from build123d import *

# Parameters (mm, degrees)
F0_W     = 30
F0_H     = 30
F1_DEPTH = 30
F2_R     = 25
F3_DEPTH = 1
F4_R     = 25
F4_R_2   = 15
F5_DEPTH = 30


with BuildPart() as f1:
    # F0 (on Top) → F1 (new body)
    with BuildSketch(Plane.XY):
        Rectangle(F0_W, F0_H)
    extrude(amount=F1_DEPTH)

    # F2 (on face) → F3 (join)
    with BuildSketch(Plane(origin=(0, 0, 0), x_dir=(1, 0, 0), z_dir=(0, 0, -1))):
        Circle(F2_R)
        Polygon((15, 15), (15, 0), (15, -15), (0, -15), (-15, -15), (-15, 3.9e-09), (-15, 15), (0, 15), align=None, mode=Mode.SUBTRACT)
        with BuildLine():
            ThreePointArc((0, -15), (10.6066017178, -10.6066017178), (15, 0))
            ThreePointArc((15, 0), (10.6066017178, 10.6066017178), (0, 15))
            ThreePointArc((0, 15), (-10.6066017164, 10.6066017192), (-15, 3.9e-09))
            ThreePointArc((-15, 3.9e-09), (-10.6066017192, -10.6066017164), (0, -15))
        make_face()
        with BuildLine():
            ThreePointArc((-15, 3.9e-09), (-10.6066017164, 10.6066017192), (0, 15))
            Line((0, 15), (-15, 15))
            Line((-15, 15), (-15, 3.9e-09))
        make_face()
        with BuildLine():
            ThreePointArc((0, 15), (10.6066017178, 10.6066017178), (15, 0))
            Line((15, 0), (15, 15))
            Line((15, 15), (0, 15))
        make_face()
        with BuildLine():
            Line((15, -15), (15, 0))
            ThreePointArc((15, 0), (10.6066017178, -10.6066017178), (0, -15))
            Line((0, -15), (15, -15))
        make_face()
        with BuildLine():
            Line((-15, -15), (0, -15))
            ThreePointArc((0, -15), (-10.6066017192, -10.6066017164), (-15, 3.9e-09))
            Line((-15, 3.9e-09), (-15, -15))
        make_face()
    extrude(amount=F3_DEPTH)

    # F4 (on face) → F5 (join)
    with BuildSketch(Plane(origin=(0, 0, -1), x_dir=(1, 0, 0), z_dir=(0, 0, -1))):
        Circle(F4_R)
        Circle(F4_R_2, mode=Mode.SUBTRACT)
    extrude(amount=F5_DEPTH)


solid = f1.part
Source: CAD feature listing. Evaluate the final solid. Frame: model axes, mm. A direction names the side the tool comes from. Give positions to 0.01 mm unless a question says otherwise; leave off trailing zeros. Write each loop counter-clockwise with the first axis right and the second up, starting at its lowest first coordinate (ties: lowest second). Pieces come first, ordered by that corner, then holes. Notation, with made-up numbers: M -15,69 L 42,69 A12 cw 42,74 Z; hole C 6.5,56.25 d5. An arc over 180 degrees is marked long. Return JSON: item names as keys, results as strings. Group by question number.
1) Cut plane C-C, the plane z = 12. Output: boundary loops of the cut face in (x, y).
2) Ray query, L1, parallel to X at y = 0, z = -10; L2, parallel to Z at x = -22, y = 9. Return the intervals inside material, ascending.
3) Cut plane D-D, the plane z = -9.5. Output: boundary loops of the cut face in (x, y), then the cut area to 3 significant figures.
4) First-contact query: pin 1 Ø2 at (y, z) = (11, 19) entering from -X; pin 2 Ø1.5 at (y, z) = (12.5, 8.5) entering from +X; pin 3 Ø2 at (y, z) = (-15.5, -24.5) entering from +X. Flat tips, straight axial feed; report the tip coordinate or a pass-through.
5) Cut plane A-A, the plane y = 0. Output: boundary loops of the cut face in (x, z), then the cut area to 3 significant figures.
6) Draft query along X for faces 1 (the face through (-14.985, -0.66, -15.79)), 2 (the face through (15, 0, 15)), 3 (the face through (0, 16, 0)). Return one class per face: released by +X, released by -X, zero draft, split by the parting line, or undercut.
7) Set-up query: faces 4 (the face through (0, 15, 15)), 5 (the face through (0, -15, 15)), 6 (the face through (-15, 0, 15)), 7 (the face through (0, 0, -1)). Return all of +Z, -Z, +X, -X, +Y, -Y with unobstructed straight access to the full face (end or side cutting, diameter ignored); none if empty.
Data:
{
 "1": {"outline": "M -15,-15 L 15,-15 L 15,15 L -15,15 Z"},
 "2": {"L1": "x = -25 to -15, 15 to 25", "L2": "z = -31 to 0"},
 "3": {"outline": "C 0,0 d50; hole C 0,0 d30", "area": "1,260 mm²"},
 "4": {"pin 1": "stops at x = -15", "pin 2": "stops at x = 15", "pin 3": "stops at x = 20.37"},
 "5": {"outline": "M -25,-31 L -15,-31 L -15,-1 L 15,-1 L 15,-31 L 25,-31 L 25,0 L 15,0 L 15,30 L -15,30 L -15,0 L -25,0 Z", "area": "1,550 mm²"},
 "6": {"face 1": "undercut", "face 2": "released by +X", "face 3": "zero draft"},
 "7": {"face 4": "+Z, +X, -X, +Y", "face 5": "+Z, +X, -X, -Y", "face 6": "+Z, -X, +Y, -Y", "face 7": "-Z"}
}
